Check sheet for the drawn part. Datum: minimum x, y, z corner. Units: mm. Round coordinates to 2 decimals unless told otherwise and drop trailing zeros. Order: outer loops, then holes, each group sorted by start corner. A loop starts at its lowest first (then second) coordinate and runs counter-clockwise, first axis right, second up.
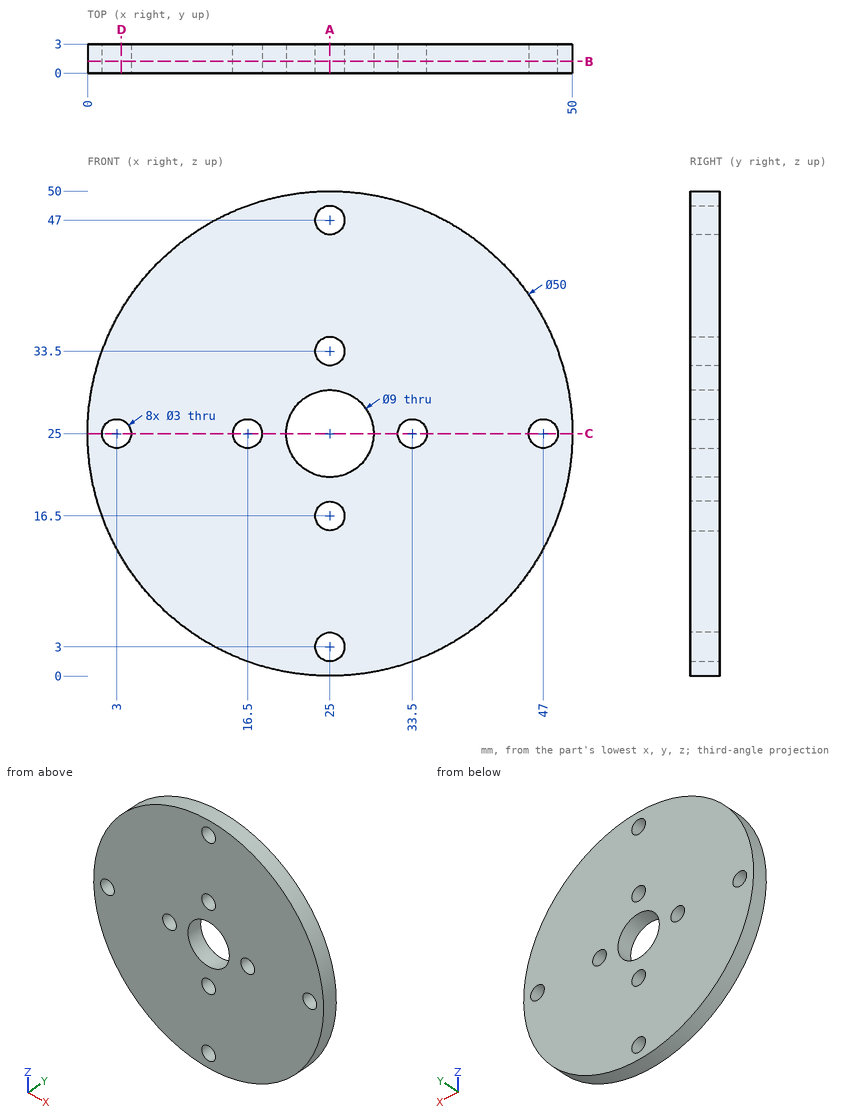
(1) Material ranges on line 1 (Z direction, x = 33.5, y = 2.35); line 2 (X direction, y = 2.5, z = 28); line 3 (X direction, y = 2.6, z = 3.5), recorded low to high.
Returned:
line 1: z = 1.49 to 23.5, 26.5 to 48.51
line 2: x = 0.18 to 21.65, 28.35 to 49.82
line 3: x = 12.24 to 23.59, 26.41 to 37.76
(2) Sectioned sample at B-B, the plane y = 1.2. Give the number of separate pieces and of enclosed holes in the cut face, and give its area (3 significant figures).
Returned:
separate pieces: 1
enclosed holes: 9
area: 1,840 mm2
(3) Sectioned sample at A-A, the plane x = 25. Record the cut outline in (y, z).
Returned:
outline: (0, 0) - (3, 0) - (3, 1.5) - (0, 1.5) - close; (0, 4.5) - (3, 4.5) - (3, 15) - (0, 15) - close; (0, 18) - (3, 18) - (3, 20.5) - (0, 20.5) - close; (0, 29.5) - (3, 29.5) - (3, 32) - (0, 32) - close; (0, 35) - (3, 35) - (3, 45.5) - (0, 45.5) - close; (0, 48.5) - (3, 48.5) - (3, 50) - (0, 50) - close
(4) Sectioned sample at D-D, the plane x = 3.5. Record the cut outline in (y, z), and give its area (3 significant figures).
Returned:
outline: (0, 12.24) - (3, 12.24) - (3, 23.59) - (0, 23.59) - close; (0, 26.41) - (3, 26.41) - (3, 37.76) - (0, 37.76) - close
area: 68.1 mm2
(5) Sectioned sample at C-C, the plane z = 25. Record the cut outline in (x, y), and give its area (3 significant figures).
Returned:
outline: (0, 0) - (1.5, 0) - (1.5, 3) - (0, 3) - close; (4.5, 0) - (15, 0) - (15, 3) - (4.5, 3) - close; (18, 0) - (20.5, 0) - (20.5, 3) - (18, 3) - close; (29.5, 0) - (32, 0) - (32, 3) - (29.5, 3) - close; (35, 0) - (45.5, 0) - (45.5, 3) - (35, 3) - close; (48.5, 0) - (50, 0) - (50, 3) - (48.5, 3) - close
area: 87.0 mm2
(6) Depth check by flat-ended pin: P1, Ø1.8, axis at x = 3, z = 25, coming from the -Y side. Enter the tip coordinate at first touch or a pass-through.
Returned:
P1: passes through
